Here's how the part is built. I have some questions about the finished solid (model axes, mm). Face numbers are marked on the shaded views. A direction names the side the tool comes from. Give positions to 0.01 mm unless a question says otherwise; leave off trailing zeros. Loops run counter-clockwise (first coordinate to the right, second up) from the corner with the lowest first, then second, coordinate; pieces in that order, holes last.
Q1. For the marked faces 1, 2 and 3, which set-ups out of +Z, -Z, +X, -X, +Y, -Y let a thin tool reach every point of the face, with its end or its side?
Q2. I need wall thicknesses on probe 1 along Y at (x, z) = (-5, 9.75); probe 2 along Z at (x, y) = (5.5, 4.25); probe 3 along X at (y, z) = (10.75, 11.5). Which ranges of each line are inside material? Lowest first, please.
Q3. I'm going to push flat-ended pins straight in: P1, Ø0.8, axis at y = -2, z = 7, coming from the +X side; P2, Ø0.5, axis at y = -2, z = -8, coming from the +X side; P3, Ø1.5, axis at x = 11, z = 8, coming from the -Y side. Where does each tip first touch, or does it pass through?
Q4. Suppose I cut it at D-D (x = -5). List the corners of the cut face in (y, z) for me, and give its area (3 significant figures).
Q5. Suppose I cut it at C-C (z = 10.75). List the corners of the cut face in (x, y) for me, and give its area (4 significant figures).
Q6. Suppose I cut it at A-A (y = 14). List the corners of the cut face in (x, z) for me.
Q7. Suppose I cut it at B-B (x = -10). List the corners of the cut face in (y, z) for me, and give its area (4 significant figures).
```python
from build123d import *

# Parameters (mm, degrees)
EXTRUDE_1_DEPTH = 19
SKETCH_2_W      = 1
SKETCH_2_H      = 1
EXTRUDE_2_DEPTH = 3.5


with BuildPart() as part:
    # 草图1 → 拉伸1 (new body)
    with BuildSketch(Plane(origin=(0, 0, 0), x_dir=(1, 0, 0), z_dir=(0, 1, 0))):
        Polygon((5, 10), (19, 10), (19, -10), (0, -10), (0, -15), (-12.5, -15), (-12.5, 12), (5, 12), align=None)
    extrude(amount=EXTRUDE_1_DEPTH)

    # 草图2 → 拉伸2 (add)
    with BuildSketch(Plane.XZ):
        with Locations((13.831603364, -8.022376545)):
            Rectangle(SKETCH_2_W, SKETCH_2_H)
        with Locations((14.016943938, 6.726433021)):
            Rectangle(SKETCH_2_W, SKETCH_2_H)
        with Locations((-6.96, 12.382327248)):
            Rectangle(SKETCH_2_W, SKETCH_2_H)
        with Locations((-1.289220796, -9.277739781)):
            Rectangle(SKETCH_2_W, SKETCH_2_H)
        with Locations((-9.959378068, -9.338614045)):
            Rectangle(SKETCH_2_W, SKETCH_2_H)
    extrude(amount=EXTRUDE_2_DEPTH)


solid = part.part
```
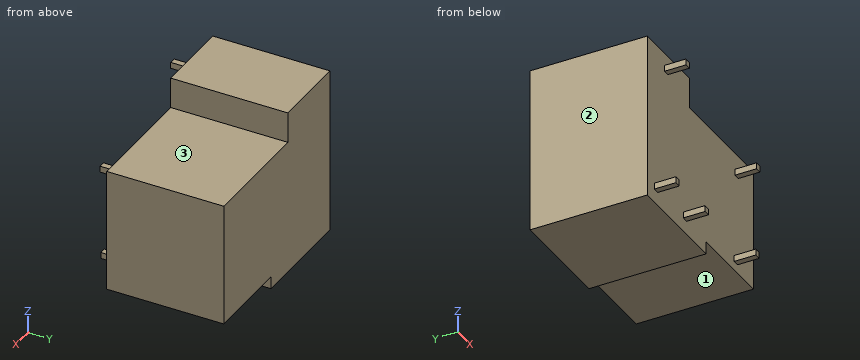
Solutions:
1. face 1: -Z, +X, +Y, -Y
1. face 2: +Z, -Z, -X, +Y, -Y
1. face 3: +Z, +X, +Y, -Y
2. probe 1: y = 0 to 19
2. probe 2: z = -10 to 10
2. probe 3: x = -12.5 to 0
3. P1: stops at x = 14.52
3. P2: stops at x = 14.33
3. P3: stops at y = 0
4. outline: (0, -12) - (19, -12) - (19, 15) - (0, 15) - close
4. area: 513 mm2
5. outline: (-12.5, 0) - (0, 0) - (0, 19) - (-12.5, 19) - close
5. area: 237.5 mm2
6. outline: (-12.5, -12) - (5, -12) - (5, -10) - (19, -10) - (19, 10) - (0, 10) - (0, 15) - (-12.5, 15) - close
7. outline: (-3.5, -9.84) - (0, -9.84) - (0, -12) - (19, -12) - (19, 15) - (0, 15) - (0, -8.84) - (-3.5, -8.84) - close
7. area: 516.5 mm2
